Drawing for the job (mm, zero at the part's lowest x, y, z). Round coordinates to 2 decimals unless told otherwise and drop trailing zeros. Write each loop counter-clockwise with the first axis right and the second up, starting at its lowest first coordinate (ties: lowest second). Pieces come first, ordered by that corner, then holes. Notation, with made-up numbers: (49.5, 46.5) - (67.5, 46.5) arc R18 ccw to (67.5, 50.5) - close; hole circle Ø3 at (33.5, 1). An arc over 180 degrees is marked (long way). One line per question, with ' | ' between items.
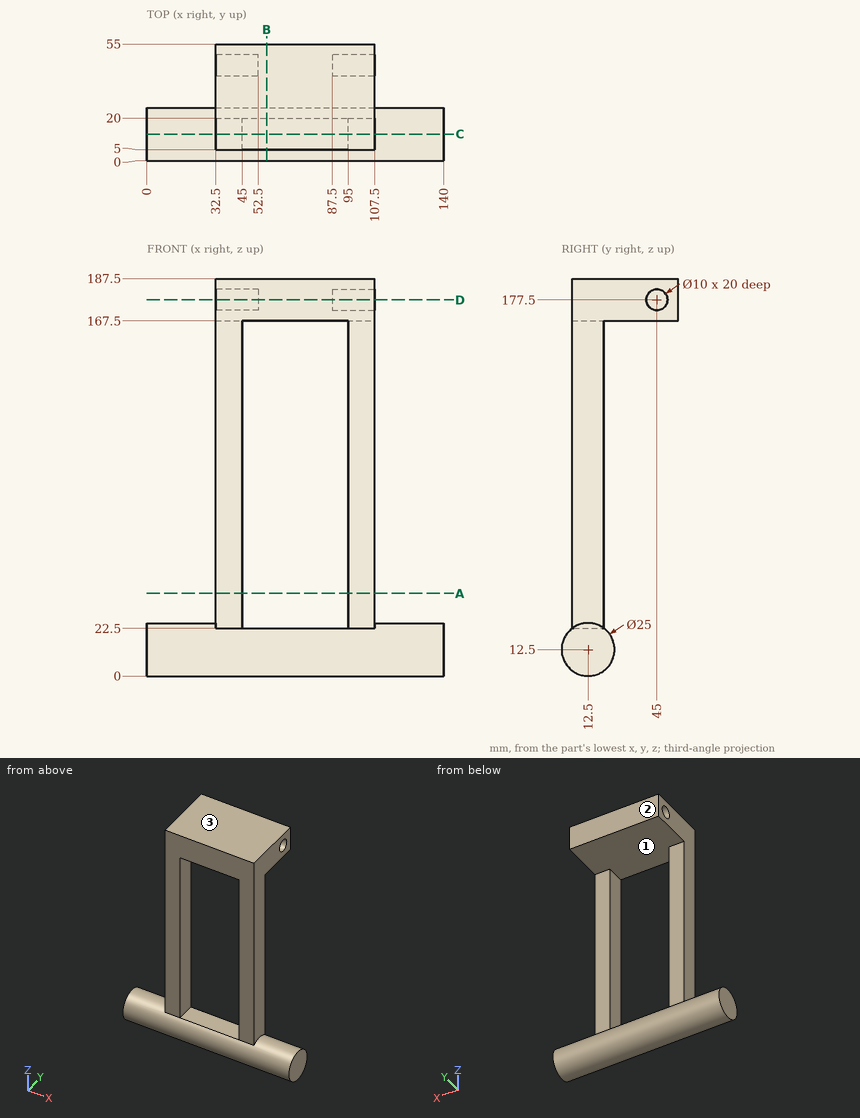
Q1. Saw through at C-C, the plane y = 12.5. List the corners of the cut face in (x, z), then the cut area to 3 significant figures.
Found:
outline: (0, 0) - (140, 0) - (140, 25) - (107.5, 25) - (107.5, 187.5) - (32.5, 187.5) - (32.5, 25) - (0, 25) - close; hole (45, 22.5) - (95, 22.5) - (95, 167.5) - (45, 167.5) - close | area: 8,440 mm^2
Q2. Saw through at B-B, the plane x = 56.5. List the corners of the cut face in (y, z).
Found:
outline: (5, 22.5) arc R12.5 ccw (long way) to (20, 22.5) - close; (5, 167.5) - (55, 167.5) - (55, 187.5) - (5, 187.5) - close
Q3. Drop flat-ended pins along their axis: pin 1 (25 mm diameter, centred on y = 32, z = 101.5, fed in from -X); pin 2 (12 mm diameter, centred on y = 12.5, z = 67, fed in from +X); pin 3 (14 mm diameter, centred on x = 38.5, z = 80.5, fed in from +Y). Give the stop position or say it passes through.
Found:
pin 1: x = 32.5 | pin 2: x = 107.5 | pin 3: y = 20
Q4. Saw through at A-A, the plane z = 39. List the corners of the cut face in (x, y), then the cut area to 3 significant figures.
Found:
outline: (32.5, 5) - (45, 5) - (45, 20) - (32.5, 20) - close; (95, 5) - (107.5, 5) - (107.5, 20) - (95, 20) - close | area: 375 mm^2
Q5. Drill centre lines: L1, parallel to Z at x = 93, y = 45; L2, parallel to X at y = 7, z = 153; L3, parallel to Y at x = 93, z = 177. Where is each one in solid material? Low to high. Write a range as from..to.
Found:
L1: 167.5..172.5, 182.5..187.5 | L2: 32.5..45, 95..107.5 | L3: 5..40.03, 49.97..55
Q6. Pull direction Z, two halves, no side cores. Call the marked faces 1, 2 and 3: +Z half, -Z half, draft (parallel to the pull), parting line (faces both ways), or undercut.
Found:
face 1: undercut | face 2: draft | face 3: +Z half
Q7. Saw through at D-D, the plane z = 177.5. List the corners of the cut face in (x, y), then the cut area to 3 significant figures.
Found:
outline: (32.5, 5) - (107.5, 5) - (107.5, 40) - (87.5, 40) - (87.5, 50) - (107.5, 50) - (107.5, 55) - (32.5, 55) - (32.5, 50) - (52.5, 50) - (52.5, 40) - (32.5, 40) - close | area: 3,350 mm^2
